Part print with two shaded views. Sizes in mm from the minimum x, y, z corner. A direction names the side the tool comes from. Coordinates: 2 decimals unless noted, no trailing zeros. Loops run counter-clockwise (first coordinate to the right, second up) from the corner with the lowest first, then second, coordinate; pieces in that order, holes last. Notation, with made-up numbers: (65, 10.5) -> (95, 10.5) arc R30 ccw to (95, 41.5) -> close; hole circle Ø10 at (89, 9). An arc over 180 degrees is marked (long way). Write each question's results on one line, items separated by ' | '.
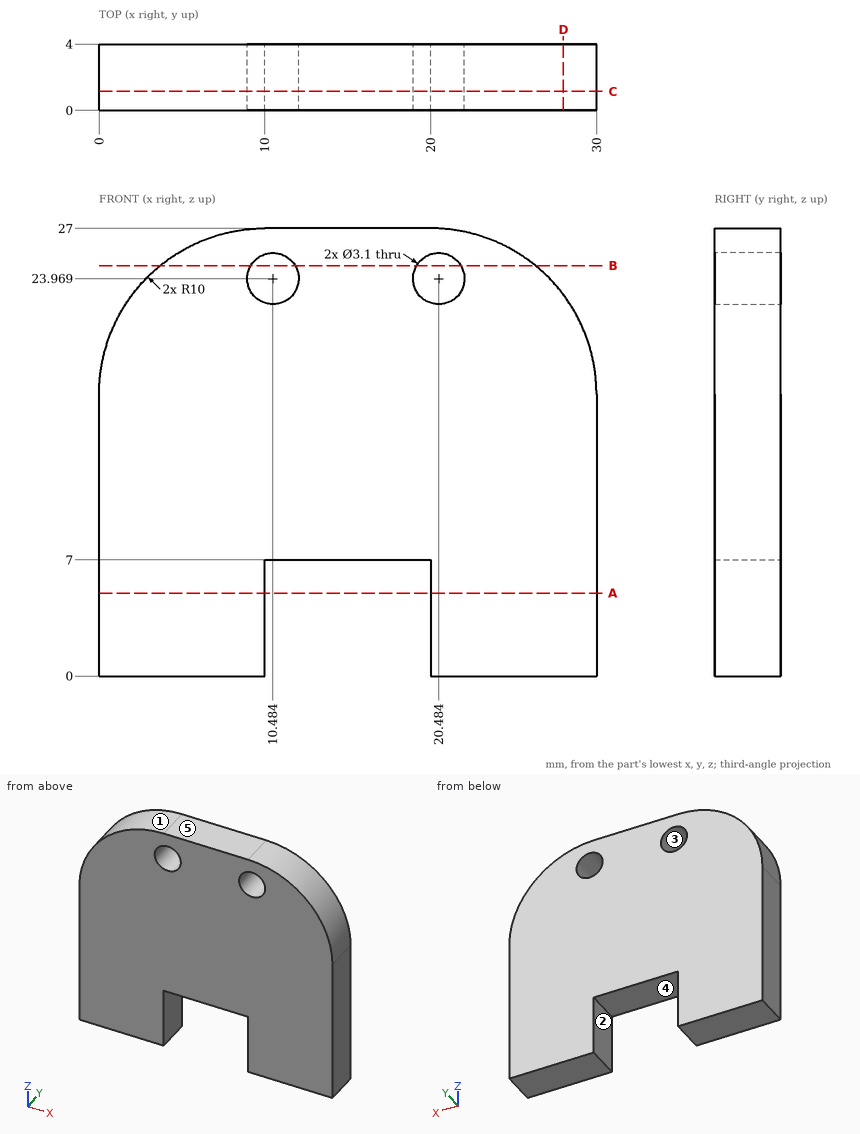
Q1. Cut at A-A on z = 5. Write the cut outline in (x, y).
Results are:
outline: (0, 0) -> (10, 0) -> (10, 4) -> (0, 4) -> close; (20, 0) -> (30, 0) -> (30, 4) -> (20, 4) -> close
Q2. Drop flat-ended pins along their axis: pin 1 (3 mm diameter, centred on x = 10.48, z = 23.97, fed in from -Y); pin 2 (1.2 mm diameter, centred on x = 13.5, y = 2.5, fed in from -Z). Give the stop position or say it passes through.
Results are:
pin 1: through | pin 2: z = 7
Q3. Cut at D-D on x = 28. Write the cut outline in (y, z).
Results are:
outline: (0, 0) -> (4, 0) -> (4, 23) -> (0, 23) -> close
Q4. Cut at B-B on z = 24.75. Write the cut outline in (x, y) (1 decimal).
Results are:
outline: (3.7, 0) -> (9.1, 0) -> (9.1, 4) -> (3.7, 4) -> close; (11.8, 0) -> (19.1, 0) -> (19.1, 4) -> (11.8, 4) -> close; (21.8, 0) -> (26.3, 0) -> (26.3, 4) -> (21.8, 4) -> close
Q5. Which spindle directions (+Z, -Z, +X, -X, +Y, -Y) get a long thin tool onto all of the face, cutting with end or side? Do the marked faces 4 and 5. Say none if no direction does.
Results are:
face 4: -Z, +Y, -Y | face 5: +Z, +X, -X, +Y, -Y
Q6. Cut at C-C on y = 1.15. Write the cut outline in (x, z).
Results are:
outline: (0, 0) -> (10, 0) -> (10, 7) -> (20, 7) -> (20, 0) -> (30, 0) -> (30, 17) arc R10 ccw to (20, 27) -> (10, 27) arc R10 ccw to (0, 17) -> close; hole circle Ø3.1 at (10.48, 23.97); hole circle Ø3.1 at (20.48, 23.97)
Q7. Wall check: L1, parallel to X at y = 0.5, z = 3.25; L2, parallel to Z at x = 18.5, y = 2.8; L3, parallel to Z at x = 9.5, y = 2.05 (1 decimal). Give the ranges that are in metal, low to high. Write a range as from..to.
Results are:
L1: 0..10, 20..30 | L2: 7..27 | L3: 0..22.8, 25.2..27
Q8. Pull direction Z, two halves, no side cores. Call the marked faces 1, 2 and 3: +Z half, -Z half, draft (parallel to the pull), parting line (faces both ways), or undercut.
Results are:
face 1: +Z half | face 2: draft | face 3: undercut
